Geometry: final body of the model. Coordinates: model frame, mm. A direction names the side the tool comes from. Give positions to 0.01 mm unless a question says otherwise; leave off trailing zeros. Write each loop counter-clockwise with the first axis right and the second up, starting at its lowest first coordinate (ties: lowest second). Pieces come first, ordered by that corner, then holes. Notation, with made-up numbers: M -33,50 L -9,50 A21 cw -9,55 Z; hole C 75.25,48 d4. An arc over 180 degrees is marked long. Answer as a JSON object with one key per item and string values.
Solid Edge part; units mm, degrees
sketch "Sketch1" plane through (0, 0, 1.016) normal (0, 0, 1) x (1, 0, 0)
  line L0 (-0.9256, 4.7235) -> (1.7124, 14.7466)
  line L1 (1.7124, 14.7466) -> (-1.0114, 26.7246)
  line L2 (-1.0114, 26.7246) -> (-5.1593, 27.4261)
  line L3 (-4.8437, 17.5537) -> (-5.1593, 27.4261)
  line L4 (-7.642, 9.3453) -> (-4.8437, 17.5537)
  line L5 (-7.642, 9.3453) -> (-14.4851, 5.5865)
  line L6 (-14.4851, 5.5865) -> (-19.1259, 5.3116)
  line L7 (-19.1259, 5.3116) -> (-27.3787, 8.9338)
  line L8 (-27.3787, 8.9338) -> (-30.0174, 12.8462)
  line L9 (-30.0174, 12.8462) -> (-37.7029, 22.3995)
  line L10 (-37.7029, 22.3995) -> (-42.4186, 19.0311)
  line L11 (-42.4186, 19.0311) -> (-36.0653, 8.2993)
  line L12 (-36.0653, 8.2993) -> (-32.8868, 3.0901)
  line L13 (-32.8868, 3.0901) -> (-30.071, 0.1266)
  line L14 (-30.071, 0.1266) -> (-20.0462, -0.5049)
  line L15 (-20.0462, -0.5049) -> (-10.6994, -0.3245)
  line L16 (-10.6994, -0.3245) -> (-4.3689, -0.3091)
  line L17 (-4.3689, -0.3091) -> (-0.9256, 4.7235)
extrude "Protrusion1" add sketch "Sketch1" along normal up to vertex (30.5976 mm away)
1) Contact query for flat-ended pins moving along their axis: P1, Ø12, axis at x = -25.5, z = 24, coming from the +Y side; P2, Ø4, axis at x = -35, z = 18.5, coming from the +Y side; P3, Ø10, axis at y = 4.5, z = 14, coming from the +X side; P4, Ø12, axis at y = 12, z = 9, coming from the +X side. Output: stop coordinate, or through.
Geometry check:
{"P1": "stops at y = 14.69", "P2": "stops at y = 21.53", "P3": "stops at x = 0.33", "P4": "stops at x = 1.71"}
2) Cut plane A-A on y = 15.5. Return loops of the section in (x, z), and give its area (3 significant figures).
Geometry check:
{"outline": "M -40.33,1.02 L -32.15,1.02 L -32.15,31.61 L -40.33,31.61 Z; M -5.54,1.02 L 1.54,1.02 L 1.54,31.61 L -5.54,31.61 Z", "area": "467 mm2"}
3) Pull-direction query (X, two-part tool) for faces 3 (the flat face through (0.37, 20.65, 16.1)), 4 (the flat face through (-16, 4, 31.614)), 5 (the flat face through (-39.286, 13.74, 16.101)), 6 (the flat face through (-6.262, 13.392, 16.101)); classes: pulls with the +X half, pulls with the -X half, needs draft (parallel to the pull), parting line crosses it, or undercut.
Geometry check:
{"face 3": "pulls with the +X half", "face 4": "needs draft", "face 5": "pulls with the -X half", "face 6": "undercut"}
4) Line query: line 1 (X direction, y = 14, z = 26.5); line 2 (X direction, y = 11.5, z = 6.5); line 3 (Y direction, x = -15.5, z = 9.5). Output: solid intervals per line, ascending. Write a range as from..to.
Geometry check:
{"line 1": "x = -39.44..-30.95, -6.06..1.52", "line 2": "x = -37.96..-29.11, -6.91..0.86", "line 3": "y = -0.42..5.53"}
5) Cut plane D-D on x = -33.5. Return loops of the section in (y, z).
Geometry check:
{"outline": "M 4.1,1.02 L 17.18,1.02 L 17.18,31.61 L 4.1,31.61 Z"}
6) Set-up query: faces 1 (the flat face through (0.375, 9.665, 16.101)), 2 (the flat face through (-28.68, 10.86, 16.1)). Return all of +Z, -Z, +X, -X, +Y, -Y with unobstructed straight access to the full face (end or side cutting, diameter ignored); none if empty.
Geometry check:
{"face 1": "+Z, -Z, +X, -Y", "face 2": "+Z, -Z, +Y"}
7) Cut plane C-C on y = 21. Return loops of the section in (x, z).
Geometry check:
{"outline": "M -39.66,1.02 L -36.58,1.02 L -36.58,31.61 L -39.66,31.61 Z; M -4.95,1.02 L 0.29,1.02 L 0.29,31.61 L -4.95,31.61 Z"}
8) Cut plane B-B on z = 21. Return loops of the section in (x, y), and give its area (3 significant figures).
Geometry check:
{"outline": "M -42.42,19.03 L -36.07,8.3 L -32.89,3.09 L -30.07,0.13 L -20.05,-0.5 L -10.7,-0.32 L -4.37,-0.31 L -0.93,4.72 L 1.71,14.75 L -1.01,26.72 L -5.16,27.43 L -4.84,17.55 L -7.64,9.35 L -14.49,5.59 L -19.13,5.31 L -27.38,8.93 L -30.02,12.85 L -37.7,22.4 Z", "area": "461 mm2"}
